```python
from build123d import *

# Parameters (mm, degrees)
SKETCH4_R       = 38.1
BASE_DEPTH      = 53.34
SKETCH5_W       = 177.8
SKETCH5_H       = 20.32
SKETCH5_H_2     = 33.02
SIDE_CUTS_DEPTH = 178.8
BOTTOM_FILLET_R = 25.4


with BuildPart() as part:
    # Sketch4 → Base (new body)
    with BuildSketch(Plane.XY):
        Polygon((38.1, -71.12), (-38.1, -71.12), (-63.5, -45.72), (-63.5, 55.88), (-12.7, 106.68), (965.2, 106.68), (1016, 55.88), (1016, -45.72), (990.6, -71.12), (914.4, -71.12), (800.1, 43.18), (152.4, 43.18), align=None)
        Circle(SKETCH4_R, mode=Mode.SUBTRACT)
        with Locations((952.5, 0)):
            Circle(SKETCH4_R, mode=Mode.SUBTRACT)
    extrude(amount=BASE_DEPTH)

    # Sketch5 → side cuts (cut, through all)
    with BuildSketch(Plane(origin=(0, 106.68, 0), x_dir=(1, 0, 0), z_dir=(0, 1, 0))):
        with Locations((25.4, -10.16)):
            Rectangle(SKETCH5_W, SKETCH5_H)
        with Locations((927.1, -36.83)):
            Rectangle(SKETCH5_W, SKETCH5_H_2)
    extrude(amount=-SIDE_CUTS_DEPTH, mode=Mode.SUBTRACT)

    # bottom fillet
    bottom_fillet_edges = [part.edges().sort_by_distance(p)[0] for p in [
        (800.1, 43.18, 26.67),
        (152.4, 43.18, 26.67),
    ]]
    fillet(bottom_fillet_edges, radius=BOTTOM_FILLET_R)


solid = part.part
```
Geometry: final body of the model. Coordinates: model frame, mm. A direction names the side the tool comes from. Round coordinates to 2 decimals unless told otherwise and drop trailing zeros. Write each loop counter-clockwise with the first axis right and the second up, starting at its lowest first coordinate (ties: lowest second). Pieces come first, ordered by that corner, then holes. Notation, with made-up numbers: (56.5, 30.25) -> (77.5, 30.25) arc R10 ccw to (77.5, 44.25) -> close; hole circle Ø6 at (-19, 22.5). An arc over 180 degrees is marked (long way). Return JSON: item names as keys, results as strings.
Q1. Section D-D on y = -9. Return the cut outline in (x, z), and give its area (3 significant figures).
From the geometry:
{"outline": "(-63.5, 20.32) -> (-37.02, 20.32) -> (-37.02, 53.34) -> (-63.5, 53.34) -> close; (37.02, 20.32) -> (100.22, 20.32) -> (100.22, 53.34) -> (37.02, 53.34) -> close; (852.28, 0) -> (915.48, 0) -> (915.48, 20.32) -> (852.28, 20.32) -> close; (989.52, 0) -> (1016, 0) -> (1016, 20.32) -> (989.52, 20.32) -> close", "area": "4,780 mm2"}
Q2. First-contact query: pin 1 Ø4 at (x, z) = (391, 7.5) entering from -Y; pin 2 Ø10 at (y, z) = (61.5, 10) entering from -X. Flat tips, straight axial feed; report the tip coordinate or a pass-through.
From the geometry:
{"pin 1": "y = 43.18", "pin 2": "x = 114.3"}
Q3. Ray query, line 1 (Y direction, x = 952.5, z = 6.75); line 2 (Y direction, x = 466, z = 30.5); line 3 (X direction, y = 0, z = 22). Return the intervals inside material, ascending.
From the geometry:
{"line 1": "-71.12 to -38.1, 38.1 to 106.68", "line 2": "43.18 to 106.68", "line 3": "-63.5 to -38.1, 38.1 to 109.22"}
Q4. Section C-C on z = 36.5. Return the cut outline in (x, y).
From the geometry:
{"outline": "(-63.5, -45.72) -> (-38.1, -71.12) -> (38.1, -71.12) -> (144.96, 35.74) arc R25.4 cw to (162.92, 43.18) -> (789.58, 43.18) arc R25.4 cw to (807.54, 35.74) -> (838.2, 5.08) -> (838.2, 106.68) -> (-12.7, 106.68) -> (-63.5, 55.88) -> close; hole circle Ø76.2 at (0, 0)"}
Q5. Set-up query: faces 1 (the flat face through (838.2, 57, 37)), 2 (the flat face through (114.3, 57, 10)), 3 (the cylindrical face through (799.17, 41.3, 27.04)), 4 (the flat face through (1, -71.12, 37)). Return all of +Z, -Z, +X, -X, +Y, -Y with unobstructed straight access to the full face (end or side cutting, diameter ignored); none if empty.
From the geometry:
{"face 1": "+Z, +X, +Y, -Y", "face 2": "-Z, -X, +Y, -Y", "face 3": "+Z, -Z, -Y", "face 4": "+Z, -Z, +X, -X, -Y"}
Q6. Section B-B on y = -58.5. Return the cut outline in (x, z).
From the geometry:
{"outline": "(-50.72, 20.32) -> (50.72, 20.32) -> (50.72, 53.34) -> (-50.72, 53.34) -> close; (901.78, 0) -> (1003.22, 0) -> (1003.22, 20.32) -> (901.78, 20.32) -> close"}
Q7. Section A-A on x = 0. Return the cut outline in (y, z).
From the geometry:
{"outline": "(-71.12, 20.32) -> (-38.1, 20.32) -> (-38.1, 53.34) -> (-71.12, 53.34) -> close; (38.1, 20.32) -> (106.68, 20.32) -> (106.68, 53.34) -> (38.1, 53.34) -> close"}
Q8. Mould query, pull axis X, two halves, no side actions, for faces 5 (the flat face through (24, 39, 20.32)), 6 (the flat face through (92.28, -16.94, 32.22)), 7 (the flat face through (990.24, 81.64, 10.02)), 8 (the cylindrical face through (153.07, 41.19, 27.04)). Classes: +X half, -X half, draft (parallel to the pull), parting line (faces both ways), or undercut.
From the geometry:
{"face 5": "draft", "face 6": "undercut", "face 7": "+X half", "face 8": "undercut"}
